Part model, mm, in its own coordinate system. A direction names the side the tool comes from. Give positions to 0.01 mm unless a question says otherwise; leave off trailing zeros. Order: outer loops, then holes, each group sorted by start corner. A loop starts at its lowest first (then second) coordinate and runs counter-clockwise, first axis right, second up. Notation, with made-up numbers: (39.25, -15.75) -> (65.25, -15.75) arc R19 cw to (65.25, 18.25) -> close; hole circle Ø9 at (28, 14.25). An arc over 180 degrees is marked (long way). Write item = value, one per line. Start each with the question number.
(1) Probe line 1 along Y through (x, z) = (27.5, 2.1); line 2 along Y through (x, z) = (47.5, 3.1); line 3 along Y through (x, z) = (30.5, 1.4). List the from-to ranges inside material, lowest first. Write a range as from..to.
(2) Saw through at C-C, the plane y = 49. List the corners of the cut face in (x, z).
(3) Two-plate mould, pull along X, no slides. Class faces 5 (the cylindrical face through (34.59, 73.6, 1.58)), 6 (the cylindrical face through (30.96, 22.594, 1.578)), 7 (the flat face through (59, 0, 2)): pulls with the +X half, pulls with the -X half, needs draft (parallel to the pull), parting line crosses it, or undercut.
(4) Flat gauge pins, fed straight in: pin 1 (1 mm diameter, centred on x = 9, z = 1.5, fed in from +Y); pin 2 (2.5 mm diameter, centred on x = 79.75, y = 23.91, fed in from +Z); pin 3 (10 mm diameter, centred on x = 73.5, y = 37, fed in from -Z); pin 4 (1.6 mm diameter, centred on y = 55.5, z = 2, fed in from +X). Where does each tip first touch, or does it go through?
(5) Which spindle directions (+Z, -Z, +X, -X, +Y, -Y) get a long thin tool onto all of the face, cutting with end or side? Do faces 1 (the flat face through (59, 30, 3.2)), 2 (the flat face through (8, 37.816, 2)), 3 (the flat face through (81, 37.816, 2)), 4 (the flat face through (26.099, 71, 2)). Say none if no direction does.
(6) Saw through at A-A, the plane x = 91. List the corners of the cut face in (y, z).
(7) Saw through at B-B, the plane z = 0.55. State how many separate pieces and enclosed holes the cut face has, then the cut area to 3 significant figures.
from build123d import *

# Parameters (mm, degrees)
SKETCH1_R           = 3.429
SKETCH1_R_2         = 2.54
BOSS_EXTRUDE1_DEPTH = 3.2004
SKETCH5_R           = 2.159
SKETCH5_W           = 40.894
SKETCH5_H           = 20.32
CUT_EXTRUDE3_DEPTH  = 4.2004
CUT_EXTRUDE4_DEPTH  = 3.2004
CUT_EXTRUDE5_DEPTH  = 3.2004
SKETCH9_W           = 2.54
SKETCH9_H           = 3.81
BOSS_EXTRUDE2_DEPTH = 3.2004
FILLET1_R           = 2.54


with BuildPart() as part:
    # Sketch1 → Boss-Extrude1 (new body)
    with BuildSketch(Plane.XY):
        with BuildLine():
            Line((120.015, 37.81552), (0, 37.81552))
            ThreePointArc((0, 37.81552), (-18.90776, 18.90776), (0, 0))
            Line((0, 0), (120.015, 0))
            ThreePointArc((120.015, 0), (138.92276, 18.90776), (120.015, 37.81552))
        make_face()
        with Locations((120.015, 18.90776)):
            Circle(SKETCH1_R, mode=Mode.SUBTRACT)
        with Locations((0, 18.90776)):
            Circle(SKETCH1_R_2, mode=Mode.SUBTRACT)
    extrude(amount=BOSS_EXTRUDE1_DEPTH)

    # Sketch5 → Cut-Extrude3 (cut, through all)
    with BuildSketch(Plane(origin=(0, 0, 0), x_dir=(-1, 0, 0), z_dir=(0, 0, -1))):
        with Locations((-79.746999972, 23.90776)):
            Circle(SKETCH5_R)
        with Locations((-29.246999972, 13.90776)):
            Circle(SKETCH5_R)
        with Locations((-29.246999972, 23.90776)):
            Circle(SKETCH5_R)
        with Locations((-79.746999972, 13.90776)):
            Circle(SKETCH5_R)
        with Locations((-54.496999972, 18.90776)):
            Rectangle(SKETCH5_W, SKETCH5_H)
    extrude(amount=-CUT_EXTRUDE3_DEPTH, mode=Mode.SUBTRACT)

    # Sketch6 → Cut-Extrude4 (cut)
    with BuildSketch(Plane.XY.offset(3.2004)):
        with BuildLine():
            Line((8.649999972, 20.49526), (25.159999972, 20.49526))
            ThreePointArc((25.159999972, 20.49526), (26.747499972, 18.90776), (25.159999972, 17.32026))
            Line((25.159999972, 17.32026), (8.649999972, 17.32026))
            ThreePointArc((8.649999972, 17.32026), (7.062499972, 18.90776), (8.649999972, 20.49526))
        make_face()
    extrude(amount=-CUT_EXTRUDE4_DEPTH, mode=Mode.SUBTRACT)

    # Sketch8 → Cut-Extrude5 (cut)
    with BuildSketch(Plane.XY.offset(3.2004)):
        Polygon((34.049999972, 15.79626), (34.049999972, 22.01926), (23.264769203, 20.49526), (23.264769203, 17.32026), align=None)
    extrude(amount=-CUT_EXTRUDE5_DEPTH, mode=Mode.SUBTRACT)

    # Sketch9 → Boss-Extrude2 (add)
    with BuildSketch(Plane(origin=(0, 0, 0), x_dir=(-1, 0, 0), z_dir=(0, 0, -1))):
        with BuildLine():
            Line((-40.703500071, 37.81552), (-15.303500071, 37.81552))
            Line((-15.303500071, 37.81552), (-20.045783141, 71.118080223))
            ThreePointArc((-20.045783141, 71.118080223), (-21.383392309, 73.573639076), (-24.003000071, 74.551710005))
            Line((-24.003000071, 74.551710005), (-32.004000071, 74.551710005))
            ThreePointArc((-32.004000071, 74.551710005), (-34.623607833, 73.573639076), (-35.961217, 71.118080223))
            Line((-35.961217, 71.118080223), (-40.703500071, 37.81552))
        make_face()
        with Locations((-31.178500071, 55.533488225)):
            Rectangle(SKETCH9_W, SKETCH9_H, mode=Mode.SUBTRACT)
        with Locations((-24.828500071, 55.533488225)):
            Rectangle(SKETCH9_W, SKETCH9_H, mode=Mode.SUBTRACT)
        with Locations((-31.178500071, 70.554572711)):
            Rectangle(SKETCH9_W, SKETCH9_H, mode=Mode.SUBTRACT)
        with Locations((-24.828500071, 70.554572711)):
            Rectangle(SKETCH9_W, SKETCH9_H, mode=Mode.SUBTRACT)
    extrude(amount=-BOSS_EXTRUDE2_DEPTH)

    # Fillet1
    fillet1_edges = [part.edges().sort_by_distance(p)[0] for p in [
        (34.049999972, 22.01926, 1.6002),
        (23.264769203, 20.49526, 1.6002),
        (23.264769203, 17.32026, 1.6002),
        (34.049999972, 15.79626, 1.6002),
    ]]
    fillet(fillet1_edges, radius=FILLET1_R)


solid = part.part
Results list:
q1.line_1 = 0..12.64, 15.18..16.72, 21.09..22.64, 25.18..74.55
q1.line_2 = 0..8.75, 29.07..37.82
q1.line_3 = 0..12.15, 15.67..16.3, 21.52..22.15, 25.67..53.63, 57.44..68.65, 72.46..74.55
q2.outline = (16.9, 0) -> (39.11, 0) -> (39.11, 3.2) -> (16.9, 3.2) -> close
q3.face_5 = pulls with the +X half
q3.face_6 = undercut
q3.face_7 = needs draft
q4.pin_1 = 37.82
q4.pin_2 = through
q4.pin_3 = 0
q4.pin_4 = 38.3
q5.face_1 = +Z, +X, -X, +Y, -Y
q5.face_2 = +Z, -Z, -X, +Y
q5.face_3 = +Z, -Z, +X, +Y
q5.face_4 = +Z, -Z
q6.outline = (0, 0) -> (37.82, 0) -> (37.82, 3.2) -> (0, 3.2) -> close
q7.separate_pieces = 1
q7.enclosed_holes = 11
q7.area = 5,310 mm^2
